```python
from build123d import *

# Parameters (mm, degrees)
BOSS_EXTRUDE1_DEPTH = 25
SKETCH2_R           = 2
CUT_EXTRUDE1_DEPTH  = 50
SKETCH4_R           = 2
CUT_EXTRUDE2_DEPTH  = 50


with BuildPart() as part:
    # Sketch1 → Boss-Extrude1 (new, symmetric)
    with BuildSketch(Plane.XY):
        Polygon((0, 0), (0, 16), (12, 16), (12, 8), (8, 8), (8, 0), align=None)
    extrude(amount=BOSS_EXTRUDE1_DEPTH, both=True)

    # Sketch2 → Cut-Extrude1 (cut)
    with BuildSketch(Plane.ZY):
        with Locations((0, 4)):
            Circle(SKETCH2_R)
    extrude(amount=-CUT_EXTRUDE1_DEPTH, mode=Mode.SUBTRACT)

    # Sketch4 → Cut-Extrude2 (cut)
    with BuildSketch(Plane(origin=(0, 16, 0), x_dir=(1, 0, 0), z_dir=(0, 1, 0))):
        with Locations(Location((4, 17, 0), (0, 0, 270))):
            Circle(SKETCH4_R)
        with Locations(Location((4, -15, 0), (0, 0, 270))):
            Circle(SKETCH4_R)
    extrude(amount=-CUT_EXTRUDE2_DEPTH, mode=Mode.SUBTRACT)


solid = part.part
```
The model under review builds one solid part; all positions refer to its coordinate system, in mm. A direction names the side the tool comes from. Coordinates: 2 decimals unless noted, no trailing zeros. Write each loop counter-clockwise with the first axis right and the second up, starting at its lowest first coordinate (ties: lowest second). Pieces come first, ordered by that corner, then holes.
1) Machinability: for faces 4 (the face through (8, 7, 0)), 5 (the face through (2.8, 8.1, -18.6)), which of the approach directions +Z, -Z, +X, -X, +Y, -Y give a long, thin tool a straight path to every point of the face, cutting with its end or side? Answer none if there is none.
2) We need section A-A on z = 0. State the section outline as (x, y) points, then the cut area to 3 significant figures.
3) Clearance check with flat-ended pins moving along their axes: pin 1 Ø3 at (x, z) = (4, 15) entering from -Y; pin 2 Ø4.5 at (x, z) = (10.5, -5) entering from -Y. State where each tip first meets the part, or that it passes through.
4) We need section B-B on y = 4. State the section outline as (x, z) points, then the cut area to 3 significant figures.
5) We need section C-C on x = 3. State the section outline as (y, z) points.
6) We need section D-D on y = 12.75. State the section outline as (x, z) points, then the cut area to 3 significant figures.
7) The part is to be moulded in two halves that separate along X. For faces 1 (the face through (4, 2, 0)), 2 (the face through (2, 8, 15)), 3 (the face through (0, 8, 0)), say which applies: pulls with the +X half, pulls with the -X half, needs draft (parallel to the pull), parting line crosses it, or undercut.
8) To check wall thickness, follow probe 1 along Y at (x, z) = (4, 0); probe 2 along X at (y, z) = (12.5, -17); probe 3 along X at (y, z) = (5, 15). State the ranges of each line that lie inside material, in increasing order.
Answer list:
1. face 4: +Z, -Z, +X, -Y
1. face 5: +Y, -Y
2. outline: (0, 0) - (8, 0) - (8, 2) - (0, 2) - close; (0, 6) - (8, 6) - (8, 8) - (12, 8) - (12, 16) - (0, 16) - close
2. area: 128 mm2
3. pin 1: passes through
3. pin 2: stops at y = 8
4. outline: (0, -25) - (8, -25) - (8, -2) - (0, -2) - close; (0, 2) - (8, 2) - (8, 25) - (0, 25) - close; hole circle Ø4 at (4, -17); hole circle Ø4 at (4, 15)
4. area: 343 mm2
5. outline: (0, -25) - (16, -25) - (16, -18.73) - (0, -18.73) - close; (0, -15.27) - (16, -15.27) - (16, 13.27) - (0, 13.27) - close; (0, 16.73) - (16, 16.73) - (16, 25) - (0, 25) - close; hole circle Ø4 at (4, 0)
6. outline: (0, -25) - (12, -25) - (12, 25) - (0, 25) - close; hole circle Ø4 at (4, -17); hole circle Ø4 at (4, 15)
6. area: 575 mm2
7. face 1: needs draft
7. face 2: undercut
7. face 3: pulls with the -X half
8. probe 1: y = 0 to 2, 6 to 16
8. probe 2: x = 0 to 2, 6 to 12
8. probe 3: x = 0 to 2, 6 to 8
